Can you work these out from the drawing? Everything is in mm from the part's minimum corner. A direction names the side the tool comes from. Round coordinates to 2 decimals unless told otherwise and drop trailing zeros. Order: outer loops, then holes, each group sorted by start corner. A loop starts at its lowest first (then second) coordinate and runs counter-clockwise, first axis right, second up. Notation, with made-up numbers: (-14.75, 43.25) -> (37.25, 43.25) arc R36 cw to (37.25, 80.25) -> close; hole circle Ø9 at (59, 82.5). An arc over 180 degrees is marked (long way). One line per item, written item: value.
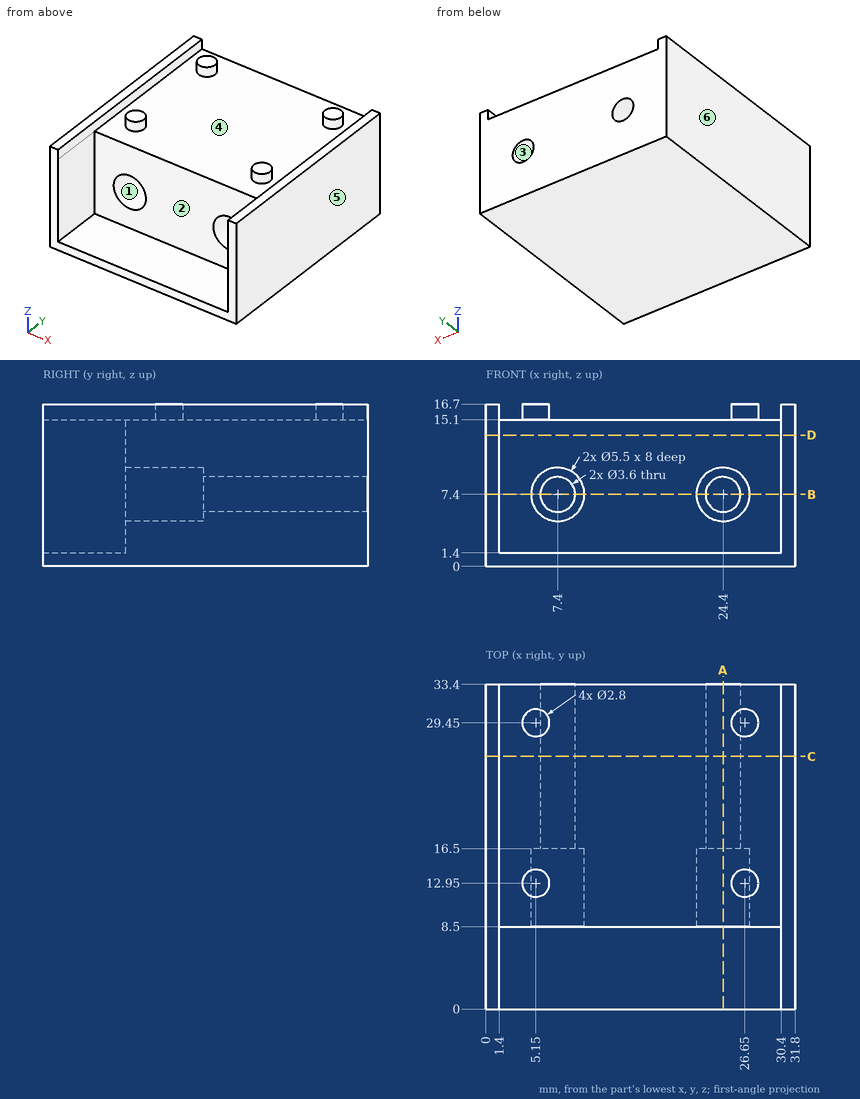
Q1. For P1, Ø7, axis at x = 18.5, z = 6.5, coming from the -Y side; P2, Ø1.6, axis at x = 7, z = 8, coming from the -Y side; P3, Ø3, axis at x = 27, y = 19, coming from the +Z side; P4, Ø1.6, axis at x = 23.5, z = 6.5, coming from the -Y side, each with a flat end and sliding along its axis, tell me the tip position at first contact or that it passes through.
Answers:
P1: y = 8.5
P2: through
P3: z = 15.1
P4: y = 16.5
Q2. Which directions (+Z, -Z, +X, -X, +Y, -Y) give clear straight access to the entire face, cutting with the end or side of a thin tool? Please do the marked faces 1, 2 and 3.
Answers:
face 1: -Y
face 2: +Z, -Y
face 3: +Y, -Y
Q3. I want a section at C-C on y = 26. Write out the boundary of the cut face in (x, z).
Answers:
outline: (0, 0) -> (31.8, 0) -> (31.8, 16.7) -> (30.4, 16.7) -> (30.4, 15.1) -> (1.4, 15.1) -> (1.4, 16.7) -> (0, 16.7) -> close; hole circle Ø3.6 at (7.4, 7.4); hole circle Ø3.6 at (24.4, 7.4)
Q4. I want a section at A-A on x = 24.4. Write out the boundary of the cut face in (y, z), then the cut area to 3 significant figures.
Answers:
outline: (0, 0) -> (33.4, 0) -> (33.4, 5.6) -> (16.5, 5.6) -> (16.5, 4.65) -> (8.5, 4.65) -> (8.5, 1.4) -> (0, 1.4) -> close; (8.5, 10.15) -> (16.5, 10.15) -> (16.5, 9.2) -> (33.4, 9.2) -> (33.4, 15.1) -> (8.5, 15.1) -> close
area: 283 mm2
Q5. If we mould it in two halves opening along X, with no side actions, what happens to the marked faces 4, 5 and 6? For each: pulls with the +X half, pulls with the -X half, needs draft (parallel to the pull), parting line crosses it, or undercut.
Answers:
face 4: undercut
face 5: pulls with the +X half
face 6: pulls with the -X half
Q6. I want a section at B-B on z = 7.4. Write out the boundary of the cut face in (x, y).
Answers:
outline: (0, 0) -> (1.4, 0) -> (1.4, 8.5) -> (4.65, 8.5) -> (4.65, 16.5) -> (5.6, 16.5) -> (5.6, 33.4) -> (0, 33.4) -> close; (9.2, 16.5) -> (10.15, 16.5) -> (10.15, 8.5) -> (21.65, 8.5) -> (21.65, 16.5) -> (22.6, 16.5) -> (22.6, 33.4) -> (9.2, 33.4) -> close; (26.2, 16.5) -> (27.15, 16.5) -> (27.15, 8.5) -> (30.4, 8.5) -> (30.4, 0) -> (31.8, 0) -> (31.8, 33.4) -> (26.2, 33.4) -> close
Q7. I want a section at D-D on z = 13.5. Write out the boundary of the cut face in (x, y), then the cut area to 3 significant figures.
Answers:
outline: (0, 0) -> (1.4, 0) -> (1.4, 8.5) -> (30.4, 8.5) -> (30.4, 0) -> (31.8, 0) -> (31.8, 33.4) -> (0, 33.4) -> close
area: 816 mm2
Q8. I need wall thicknesses on line 1 along X through (y, z) = (9.5, 8); line 2 along X through (y, z) = (21.5, 16); line 3 along Z through (x, y) = (24.4, 14). Which ranges of each line are inside material? Lowest first, please.
Answers:
line 1: 0 to 4.72, 10.08 to 21.72, 27.08 to 31.8
line 2: 0 to 1.4, 30.4 to 31.8
line 3: 0 to 4.65, 10.15 to 15.1
